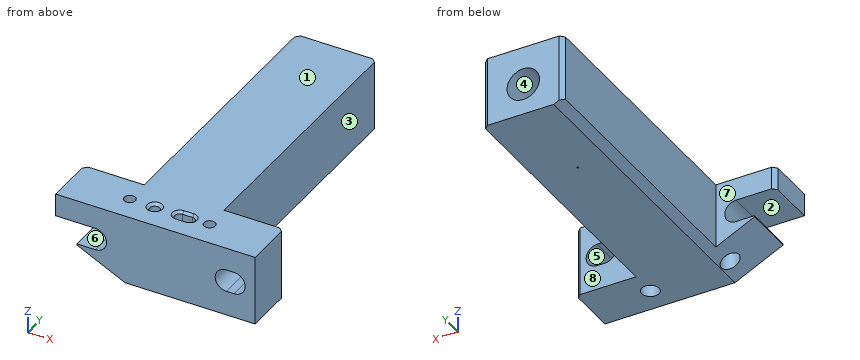
from build123d import *

# Parameters (mm, degrees)
EXTRUDE1_DEPTH                                   = 44.45
CHAMFER1_SIZE                                    = 2.54
CHAMFER2_SIZE                                    = 2.54
F_13_16_0_8125_DIAMETER_HOLE1_D                  = 20.6375
F_13_16_0_8125_DIAMETER_HOLE1_DEPTH              = 63.754
F_60_0_04_DIAMETER_HOLE1_REACH                   = 46.45
F_60_0_04_DIAMETER_HOLE1_BORE_R                  = 0.508
CBORE_FOR_1_4_SOCKET_HEAD_CAP_SCREW1_D           = 7.14248
CBORE_FOR_1_4_SOCKET_HEAD_CAP_SCREW1_CBORE_D     = 11.1125
CBORE_FOR_1_4_SOCKET_HEAD_CAP_SCREW1_CBORE_DEPTH = 15.748
F_1_4_0_25_DIAMETER_HOLE2_D                      = 6.36778
F_1_4_0_25_DIAMETER_HOLE2_DEPTH                  = 12.7
F_1_4_0_25_DIAMETER_HOLE2_CSINK_D                = 9.652
F_1_4_0_25_DIAMETER_HOLE2_CSINK_ANGLE            = 90
F_1_4_0_25_DIAMETER_HOLE2_TIP                    = 1.913074116
EXTRUDE4_DEPTH                                   = 12.7
F_1_2_20_TAPPED_HOLE3_D                          = 11.50874
F_1_2_20_TAPPED_HOLE3_DEPTH                      = 82.55
F_1_2_20_TAPPED_HOLE3_TIP                        = 3.322287069
EXTRUDE5_DEPTH                                   = 172.0690001
EXTRUDE5_DEPTH_BACK                              = 33.02
CHAMFER3_SIZE                                    = 1.524
EXTRUDE6_DEPTH                                   = 33.131
CUT_EXTRUDE1_DEPTH                               = 33.131


with BuildPart() as part:
    # Sketch1 → Extrude1 (new body)
    with BuildSketch(Plane.XY):
        Polygon((-63.5, 19.16234013), (-25.4, 19.16234013), (-25.4, 190.23134013), (0, 190.23134013), (0, -12.96865987), (-63.5, -12.96865987), align=None)
    extrude1 = extrude(amount=EXTRUDE1_DEPTH)

    # Mirror2: Extrude1 across plane
    add(extrude1.mirror(Plane(origin=(0, -12.96865987, 44.45), x_dir=(0, 0, 1), z_dir=(-1, 0, 0))))

    # Chamfer1
    chamfer1_edges = [part.edges().sort_by_distance(p)[0] for p in [
        (63.5, 19.16234013, 22.225),
        (25.4, 190.23134013, 22.225),
    ]]
    chamfer(chamfer1_edges, length=CHAMFER1_SIZE)

    # Chamfer2
    chamfer2_edges = [part.edges().sort_by_distance(p)[0] for p in [
        (-63.5, 19.16234013, 22.225),
        (-25.4, 190.23134013, 22.225),
    ]]
    chamfer(chamfer2_edges, length=CHAMFER2_SIZE)

    # 13/16 (0.8125) Diameter Hole1
    with Locations(Plane(origin=(0, 190.23134013, 19.939), x_dir=(0, 0, 1), z_dir=(0, 1, 0))):
        with Locations((0, 0)):
            Hole(F_13_16_0_8125_DIAMETER_HOLE1_D / 2, depth=F_13_16_0_8125_DIAMETER_HOLE1_DEPTH)

    # #60 (0.04) Diameter Hole1 bore → #60 (0.04) Diameter Hole1 (cut, up to next)
    with BuildSketch(Plane(origin=(0, 0, 0), x_dir=(-1, 0, 0), z_dir=(0, 0, -1)), mode=Mode.PRIVATE) as f_60_0_04_diameter_hole1_sk1:
        with Locations((0, 129.27134013)):
            Circle(F_60_0_04_DIAMETER_HOLE1_BORE_R)
    f_60_0_04_diameter_hole1_tool1 = extrude(f_60_0_04_diameter_hole1_sk1.sketch, amount=-F_60_0_04_DIAMETER_HOLE1_REACH, mode=Mode.PRIVATE) & part.part
    add(f_60_0_04_diameter_hole1_tool1.solids().sort_by_distance((0, 129.27134, 0))[0], mode=Mode.SUBTRACT)

    # CBORE for 1/4 Socket Head Cap Screw1 (through all)
    with Locations(Plane(origin=(25.4, 3.09684013, 0), x_dir=(-1, 0, 0), z_dir=(0, 0, -1))):
        with Locations((0, 0), (50.8, 0)):
            CounterBoreHole(CBORE_FOR_1_4_SOCKET_HEAD_CAP_SCREW1_D / 2, CBORE_FOR_1_4_SOCKET_HEAD_CAP_SCREW1_CBORE_D / 2, CBORE_FOR_1_4_SOCKET_HEAD_CAP_SCREW1_CBORE_DEPTH)

    # 1/4 (0.25) Diameter Hole2
    with Locations(Plane.XY.offset(44.45)):
        with Locations((-9.525, 3.09684013)):
            CounterSinkHole(F_1_4_0_25_DIAMETER_HOLE2_D / 2, F_1_4_0_25_DIAMETER_HOLE2_CSINK_D / 2, depth=F_1_4_0_25_DIAMETER_HOLE2_DEPTH, counter_sink_angle=F_1_4_0_25_DIAMETER_HOLE2_CSINK_ANGLE)
            with Locations((0, 0, -(F_1_4_0_25_DIAMETER_HOLE2_DEPTH + F_1_4_0_25_DIAMETER_HOLE2_TIP / 2))):  # 118° drill point
                Cone(0, F_1_4_0_25_DIAMETER_HOLE2_D / 2, F_1_4_0_25_DIAMETER_HOLE2_TIP, mode=Mode.SUBTRACT)

    # Sketch22 → Extrude4 (cut)
    with BuildSketch(Plane.XY.offset(44.45)):
        with BuildLine():
            Line((12.7, -0.08704987), (6.35, -0.08704987))
            ThreePointArc((6.35, -0.08704987), (3.16611, 3.09684013), (6.35, 6.28073013))
            Line((6.35, 6.28073013), (12.7, 6.28073013))
            ThreePointArc((12.7, 6.28073013), (15.88389, 3.09684013), (12.7, -0.08704987))
        make_face()
    extrude(amount=-EXTRUDE4_DEPTH, mode=Mode.SUBTRACT)

    # 1/2-20 Tapped Hole3
    with Locations(Plane(origin=(0, 126.47734013, 0), x_dir=(-1, 0, 0), z_dir=(0, 1, 0))):
        with Locations((0, 19.939)):
            Hole(F_1_2_20_TAPPED_HOLE3_D / 2, depth=F_1_2_20_TAPPED_HOLE3_DEPTH)
            with Locations((0, 0, -(F_1_2_20_TAPPED_HOLE3_DEPTH + F_1_2_20_TAPPED_HOLE3_TIP / 2))):  # 120° drill point
                Cone(0, F_1_2_20_TAPPED_HOLE3_D / 2, F_1_2_20_TAPPED_HOLE3_TIP, mode=Mode.SUBTRACT)

    # Sketch27 → Extrude5 (cut, two sides)
    with BuildSketch(Plane(origin=(0, 19.16234013, 0), x_dir=(1, 0, 0), z_dir=(0, 1, 0))) as extrude5_sk:
        Polygon((-19.338095495, 0), (-63.5, -21.5392), (-63.5, 0), align=None)
    extrude(amount=EXTRUDE5_DEPTH, mode=Mode.SUBTRACT)
    extrude(extrude5_sk.sketch, amount=-EXTRUDE5_DEPTH_BACK, mode=Mode.SUBTRACT)

    # Chamfer3
    chamfer3_edges = [part.edges().sort_by_distance(p)[0] for p in [
        (15.88389, 3.09684013, 44.45),
        (9.525, 6.28073013, 44.45),
        (3.16611, 3.09684013, 44.45),
        (9.525, -0.08704987, 44.45),
    ]]
    chamfer(chamfer3_edges, length=CHAMFER3_SIZE)

    # Sketch28 → Extrude6 (cut, through all)
    with BuildSketch(Plane(origin=(0, 19.16234013, 0), x_dir=(1, 0, 0), z_dir=(0, 1, 0))):
        with BuildLine():
            Line((45.212, -15.7226), (50.038, -15.7226))
            ThreePointArc((50.038, -15.7226), (57.1754, -22.86), (50.038, -29.9974))
            Line((50.038, -29.9974), (45.212, -29.9974))
            ThreePointArc((45.212, -29.9974), (38.0746, -22.86), (45.212, -15.7226))
        make_face()
        with BuildLine():
            Line((-38.227, -29.9974), (-63.627, -29.9974))
            ThreePointArc((-63.627, -29.9974), (-70.7644, -22.86), (-63.627, -15.7226))
            Line((-63.627, -15.7226), (-38.227, -15.7226))
            ThreePointArc((-38.227, -15.7226), (-31.0896, -22.86), (-38.227, -29.9974))
        make_face()
    extrude(amount=-EXTRUDE6_DEPTH, mode=Mode.SUBTRACT)

    # Sketch29 → Cut-Extrude1 (cut, through all)
    with BuildSketch(Plane(origin=(0, 19.16234013, 0), x_dir=(1, 0, 0), z_dir=(0, 1, 0))):
        Polygon((-51.574202675, -15.7226), (-50.050202675, -14.979295535), (-50.050202675, -15.7226), align=None)
    extrude(amount=-CUT_EXTRUDE1_DEPTH, mode=Mode.SUBTRACT)


solid = part.part
Source: CAD feature listing. Evaluate the final solid. Frame: model axes, mm. Face numbers are marked on the shaded views. A direction names the side the tool comes from. Round coordinates to 2 decimals unless told otherwise and drop trailing zeros. Order: outer loops, then holes, each group sorted by start corner. A loop starts at its lowest first (then second) coordinate and runs counter-clockwise, first axis right, second up. Notation, with made-up numbers: (54, 35) - (106, 35) arc R22 ccw to (106, 51) - close; hole circle Ø2 at (-11.75, 24.5). An arc over 180 degrees is marked (long way). Use a Markdown table: item, result. Add a question column.
1. First-contact query: pin 1 (5.5 mm diameter, centred on x = 47, y = 1, fed in from -Z); pin 2 (5.5 mm diameter, centred on x = -27, y = 1, fed in from -Z); pin 3 (3 mm diameter, centred on x = 9, y = 2.5, fed in from +Z). Flat tips, straight axial feed; report the tip coordinate or a pass-through.
2. Section query D-D (x = 42). Return the cut outline in (y, z), then the cut area to 3 significant figures.
3. Section query B-B (z = 22.86). Give the number of separate pieces and of enclosed holes in the cut face, then the cut area to 3 significant figures.
4. Set-up query: the marked faces 4, 5, 6, 7 and 8. Return all of +Z, -Z, +X, -X, +Y, -Y with unobstructed straight access to the full face (end or side cutting, diameter ignored); none if empty.
5. Line query: probe 1 along X at (y, z) = (145, 20.5); probe 2 along Y at (x, z) = (0, 5.25); probe 3 along Y at (x, z) = (-26, 5). Output: solid intervals per line, ascending.
6. Section query C-C (y = 71.5). Return the cut outline in (x, z).
7. Section query A-A (x = -34). Return the cut outline in (y, z).
8. Mould query, pull axis Z, two halves, no side actions, for the marked faces 1, 2 and 3. Classes: +Z half, -Z half, draft (parallel to the pull), parting line (faces both ways), or undercut.
Derived:
| question | item | result |
|---|---|---|
| 1 | pin 1 | z = 0 |
| 1 | pin 2 | z = 15.75 |
| 1 | pin 3 | z = 31.75 |
| 2 | outline | (-12.97, 0) - (19.16, 0) - (19.16, 16.49) - (-12.97, 16.49) - close; (-12.97, 29.23) - (19.16, 29.23) - (19.16, 44.45) - (-12.97, 44.45) - close |
| 2 | area | 1,020 mm2 |
| 3 | separate pieces | 2 |
| 3 | enclosed holes | 2 |
| 3 | area | 8,940 mm2 |
| 4 | face 4 | +Y |
| 4 | face 5 | +Y, -Y |
| 4 | face 6 | -X, +Y, -Y |
| 4 | face 7 | +Z, -Z, -X, +Y |
| 4 | face 8 | +Z, -Z, +X, +Y |
| 5 | probe 1 | -25.4 to -10.3, 10.3 to 25.4 |
| 5 | probe 2 | -12.97 to 128.76, 129.78 to 190.23 |
| 5 | probe 3 | -12.97 to -2.43, 8.62 to 19.16 |
| 6 | outline | (-25.4, 2.96) - (-19.34, 0) - (25.4, 0) - (25.4, 44.45) - (-25.4, 44.45) - close; hole circle Ø11.51 at (0, 19.94) |
| 7 | outline | (-12.97, 7.15) - (19.16, 7.15) - (19.16, 17.11) - (-12.97, 17.11) - close; (-12.97, 28.61) - (19.16, 28.61) - (19.16, 44.45) - (-12.97, 44.45) - close |
| 8 | face 1 | +Z half |
| 8 | face 2 | undercut |
| 8 | face 3 | draft |
